Source: CAD feature listing. Evaluate the final solid. Frame: model axes, mm. Round coordinates to 2 decimals unless told otherwise and drop trailing zeros. Write each loop counter-clockwise with the first axis right and the second up, starting at its lowest first coordinate (ties: lowest second). Pieces come first, ordered by that corner, then holes. Notation, with made-up numbers: M 31,-34.5 L 66,-34.5 A21 ccw 66,-30.5 Z; hole C -7,76.25 d11. An arc over 180 degrees is marked long. Use a Markdown table: item, result.
```python
from build123d import *

# Parameters (mm, degrees)
SKETCH1_R               = 2.75
BOSS_EXTRUDE1_DEPTH     = 210
CUT_EXTRUDE1_DEPTH      = 211.036008818
CUT_EXTRUDE1_DEPTH_BACK = 211.036008818
SKETCH2_R               = 1
CUT_EXTRUDE2_DEPTH      = 211.03600892
CUT_EXTRUDE2_DEPTH_BACK = 211.03600892
SKETCH3_R               = 1


with BuildPart() as part:
    # Sketch1 → Boss-Extrude1 (new body)
    with BuildSketch(Plane.XY):
        Circle(SKETCH1_R)
    extrude(amount=BOSS_EXTRUDE1_DEPTH)

    # Sketch2 → Cut-Extrude1 (cut, two sides: drawn at the far end of the back side and taken through both)
    with BuildSketch(Plane(origin=(0, 0, 0), x_dir=(1, 0, 0), z_dir=(0, 1, 0)).offset(-CUT_EXTRUDE1_DEPTH_BACK)):
        with Locations(Location((0, -5, 0), (0, 0, 270))):
            Circle(SKETCH2_R)
    extrude(amount=CUT_EXTRUDE1_DEPTH + CUT_EXTRUDE1_DEPTH_BACK, mode=Mode.SUBTRACT)

    # Sketch3 → Cut-Extrude2 (cut, two sides: drawn at the far end of the back side and taken through both)
    with BuildSketch(Plane(origin=(0, 0, 0), x_dir=(1, 0, 0), z_dir=(0, 1, 0)).offset(-CUT_EXTRUDE2_DEPTH_BACK)):
        with Locations(Location((0, -205, 0), (0, 0, 270))):
            Circle(SKETCH3_R)
    extrude(amount=CUT_EXTRUDE2_DEPTH + CUT_EXTRUDE2_DEPTH_BACK, mode=Mode.SUBTRACT)


solid = part.part
```
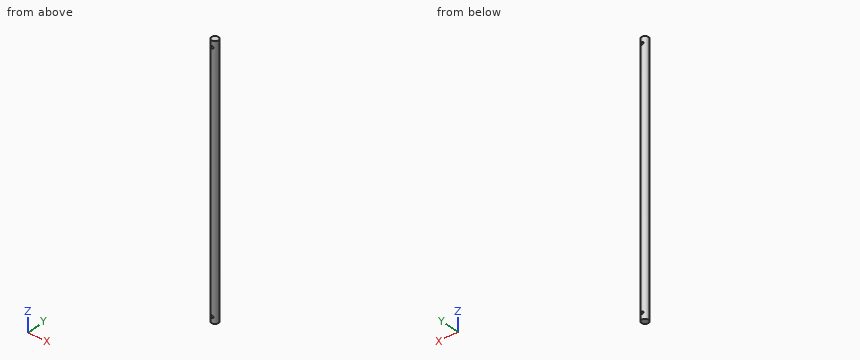
Q1. Section B-B on z = 87.5. Return loops of the section in (x, y).
Results are:
| item | result |
|---|---|
| outline | C 0,0 d5.5 |
Q2. First-contact query: pin 1 Ø2 at (y, z) = (2, 157.5) entering from -X. Flat tip, straight axial feed; report the tip coordinate or a pass-through.
Results are:
| item | result |
|---|---|
| pin 1 | x = -2.56 |
Q3. Section C-C on y = -1.25. Return loops of the section in (x, z).
Results are:
| item | result |
|---|---|
| outline | M -2.45,0 L 2.45,0 L 2.45,210 L -2.45,210 Z; hole C 0,5 d2; hole C 0,205 d2 |
Q4. Section A-A on x = 0. Return loops of the section in (y, z).
Results are:
| item | result |
|---|---|
| outline | M -2.75,0 L 2.75,0 L 2.75,4 L -2.75,4 Z; M -2.75,6 L 2.75,6 L 2.75,204 L -2.75,204 Z; M -2.75,206 L 2.75,206 L 2.75,210 L -2.75,210 Z |
Q5. Line query: L1, parallel to Z at x = 0, y = -0.5; L2, parallel to X at y = -0.4, z = 5; L3, parallel to Z at x = 0.9, y = -1.2. Output: solid intervals per line, ascending.
Results are:
| item | result |
|---|---|
| L1 | 0 to 4, 6 to 204, 206 to 210 |
| L2 | -2.72 to -1, 1 to 2.72 |
| L3 | 0 to 4.56, 5.44 to 204.56, 205.44 to 210 |
